Geometry: final body of the model. Coordinates: model frame, mm. A direction names the side the tool comes from. Coordinates: 2 decimals unless noted, no trailing zeros. Order: outer loops, then holes, each group sorted by start corner. A loop starts at its lowest first (then second) coordinate and runs counter-clockwise, first axis right, second up. Notation, with made-up numbers: (21.25, 65.25) - (63.25, 65.25) arc R16 ccw to (63.25, 83.25) - close; hole circle Ø1 at (87, -22). An arc over 180 degrees is marked (long way). Use a Markdown table: item, result. Add a question column.
Autodesk Inventor part; units mm, degrees
ref_plane "pick_place_pad_XY" through (0, 0, 0) normal (0, 1, 0) x (1, 0, 0)
ref_plane "pick_place_pad_YZ" through (0, 0, 0) normal (1, 0, 0) x (0, 0, -1)
ref_plane "pick_place_pad_ZX" through (0, 0, 0) normal (0, 0, -1) x (0, 1, 0)
sketch "Sketch_6" plane through (0, 0, 0) normal (1, 0, 0) x (0, 1, 0)
  line L0 (0, 3.175) -> (-1.27, 3.175)
  line L1 (-1.27, 3.175) -> (-1.27, 2.407)
  arc A0 (-1.397, 2.28) -> (-1.27, 2.407) centre (-1.397, 2.407) ccw
  line L2 (-1.397, 2.28) -> (-6.54, 2.28)
  arc A1 (-6.54, 2.28) -> (-6.54, 1.645) centre (-6.54, 1.9625) ccw
  line L3 (-6.54, 1.645) -> (-6.477, 1.645)
  arc A2 (-6.477, 1.645) -> (-5.715, 1.645) centre (-6.096, 2.153) ccw
  line L4 (-5.715, 1.645) -> (-1.397, 1.645)
  arc A3 (-1.27, 1.518) -> (-1.397, 1.645) centre (-1.397, 1.518) ccw
  line L5 (-1.27, 1.518) -> (-1.27, 1.022)
  arc A4 (-1.397, 0.895) -> (-1.27, 1.022) centre (-1.397, 1.022) ccw
  line L6 (-1.397, 0.895) -> (-5.715, 0.895)
  arc A5 (-5.715, 0.895) -> (-6.477, 0.895) centre (-6.096, 0.387) ccw
  line L7 (-6.477, 0.895) -> (-6.5222, 0.895)
  arc A6 (-6.5222, 0.895) -> (-6.5222, 0.26) centre (-6.5227, 0.5775) ccw
  line L8 (-6.5222, 0.26) -> (-1.397, 0.26)
  arc A7 (-1.27, 0.133) -> (-1.397, 0.26) centre (-1.397, 0.133) ccw
  line L9 (-1.27, 0.133) -> (-1.27, -0.133)
  arc A8 (-1.397, -0.26) -> (-1.27, -0.133) centre (-1.397, -0.133) ccw
  line L10 (-1.397, -0.26) -> (-6.54, -0.26)
  arc A9 (-6.54, -0.26) -> (-6.54, -0.895) centre (-6.54, -0.5775) ccw
  line L11 (-6.54, -0.895) -> (-6.477, -0.895)
  arc A10 (-6.477, -0.895) -> (-5.715, -0.895) centre (-6.096, -0.387) ccw
  line L12 (-5.715, -0.895) -> (-1.397, -0.895)
  arc A11 (-1.27, -1.022) -> (-1.397, -0.895) centre (-1.397, -1.022) ccw
  line L13 (-1.27, -1.022) -> (-1.27, -1.518)
  arc A12 (-1.397, -1.645) -> (-1.27, -1.518) centre (-1.397, -1.518) ccw
  line L14 (-1.397, -1.645) -> (-5.715, -1.645)
  arc A13 (-5.715, -1.645) -> (-6.477, -1.645) centre (-6.096, -2.153) ccw
  line L15 (-6.477, -1.645) -> (-6.54, -1.645)
  arc A14 (-6.54, -1.645) -> (-6.54, -2.28) centre (-6.54, -1.9625) ccw
  line L16 (-6.54, -2.28) -> (-1.397, -2.28)
  arc A15 (-1.27, -2.407) -> (-1.397, -2.28) centre (-1.397, -2.407) ccw
  line L17 (-1.27, -2.407) -> (-1.27, -3.175)
  line L18 (-1.27, -3.175) -> (0, -3.175)
  line L19 (0, -3.175) -> (0, 3.175)
extrude "Extrusion1" add sketch "Sketch_6" along normal mid plane 9.906
ref_plane "pick_place_pad_XY" through (0, 0, 0) normal (0, 1, 0) x (1, 0, 0)
ref_plane "pick_place_pad_YZ" through (0, 0, 0) normal (1, 0, 0) x (0, 0, -1)
ref_plane "pick_place_pad_ZX" through (0, 0, 0) normal (0, 0, -1) x (0, 1, 0)
properties part number "PPP-06-01-20--DV"
1) Section query B-B (z = 0). Return the cut outline in (x, y), and give its area (3 significant figures).
2) Line query: line 1 (Z direction, x = -0.25, y = -1.75) (3 decimals); line 2 (Z direction, x = 3.5, y = -6); line 3 (Y direction, x = -1.25, z = -2). Output: solid intervals per line, ascending. Write a range as from..to.
3) First-contact query: pin 1 (0.6 mm diameter, centred on x = -2, z = -3, fed in from -Y); pin 2 (2 mm diameter, centred on x = 3.5, z = 1, fed in from +Y); pin 3 (4 mm diameter, centred on x = 3, y = -5, fed in from -Z); pin 4 (1.3 mm diameter, centred on x = -1, y = -4, fed in from +Z). Flat tips, straight axial feed; report the tip coordinate or a pass-through.
4) Section query A-A (y = -5.5). Return the cut outline in (x, z) (3 decimals), and give its area (3 significant figures).
5) Draft query along Z for faces 4 (the flat face through (0, -4, 0.26)), 5 (the flat face through (0, -4, -1.645)), 6 (the flat face through (4.953, -2.7, -0.7)), 7 (the flat face through (0, -1, 3.175)). Return one class per face: released by +Z, released by -Z, zero draft, split by the parting line, or undercut.
6) Access query for faces 1 (the flat face through (0, -4, -0.26)), 2 (the flat face through (0, -4, 1.645)), 3 (the flat face through (0, -4, 2.28)). Directions: +Z, -Z, +X, -X, +Y, -Y. A direction counts if a zero-diameter tool reaches every point of the face in a straight line with its end or side. Return the directions, or none.
From the geometry:
| question | item | result |
|---|---|---|
| 1 | outline | (-4.95, -1.27) - (4.95, -1.27) - (4.95, 0) - (-4.95, 0) - close |
| 1 | area | 12.6 mm^2 |
| 2 | line 1 | z = -2.28..-1.645, -0.895..-0.26, 0.26..0.895, 1.645..2.28 |
| 2 | line 2 | z = -2.28..-1.53, -1.01..-0.26, 0.26..1.01, 1.53..2.28 |
| 2 | line 3 | y = -6.86..0 |
| 3 | pin 1 | stops at y = -1.27 |
| 3 | pin 2 | stops at y = 0 |
| 3 | pin 3 | stops at z = -2.28 |
| 3 | pin 4 | stops at z = 2.28 |
| 4 | outline | (-4.953, -2.28) - (4.953, -2.28) - (4.953, -1.645) - (-4.953, -1.645) - close; (-4.953, -0.895) - (4.953, -0.895) - (4.953, -0.26) - (-4.953, -0.26) - close; (-4.953, 0.26) - (4.953, 0.26) - (4.953, 0.895) - (-4.953, 0.895) - close; (-4.953, 1.645) - (4.953, 1.645) - (4.953, 2.28) - (-4.953, 2.28) - close |
| 4 | area | 25.2 mm^2 |
| 5 | face 4 | undercut |
| 5 | face 5 | undercut |
| 5 | face 6 | zero draft |
| 5 | face 7 | released by +Z |
| 6 | face 1 | +X, -X, -Y |
| 6 | face 2 | +X, -X |
| 6 | face 3 | +Z, +X, -X, -Y |
